Geometry check sheet. Reference: the model listing, model coordinates, mm. A direction names the side the tool comes from. Coordinates: 2 decimals unless noted, no trailing zeros. Write each loop counter-clockwise with the first axis right and the second up, starting at its lowest first coordinate (ties: lowest second). Pieces come first, ordered by that corner, then holes. Notation, with made-up numbers: (-35, 54) -> (16, 54) arc R21 ccw to (16, 91) -> close; hole circle Ø7 at (-36.5, 59.5). An arc over 180 degrees is marked (long way). Answer in a Markdown table with one row per item. Add a question column.
1. Set-up check for faces 4 (the cylindrical face through (-4.769, 7.888, -21.477)), 5 (the cylindrical face through (35.405, 47.707, -13.399)), 6 (the cylindrical face through (35.85, 45.21, -15.5)), 7 (the flat face through (38, 53, 14)): record each of +Z, -Z, +X, -X, +Y, -Y from which the full face is reachable in a straight line by a thin tool's end or side.
2. Cross-section at D-D on y = 68. Record the cut outline in (x, z), and give its area (3 significant figures).
3. Scan lines: L1, parallel to Y at x = 36, z = 31; L2, parallel to Z at x = 0, y = 18; L3, parallel to Y at x = -19, z = -1. Record each from-to range of solid material in increasing order. Write a range as from..to.
4. Mould release check, pull along X, two halves, no side actions. Record for faces 1 (the conical face through (-26.848, 33.914, 1.182)), 2 (the flat face through (39, 53, 17)), 3 (the flat face through (36.6, 46.6, 0.2)): pulls with the +X half, pulls with the -X half, needs draft (parallel to the pull), parting line crosses it, or undercut.
5. Cross-section at A-A on x = 0. Give the number of separate pieces and of enclosed holes in the cut face, and give its area (3 significant figures).
6. Depth check by flat-ended pin: P1, Ø6, axis at x = 34.5, y = 52, coming from the -Z side; P2, Ø5.5, axis at x = 36.5, y = 51, coming from the -Z side; P3, Ø1.5, axis at y = 59, z = -27, coming from the +X side; P4, Ø5, axis at x = -14, z = 0, coming from the -Y side. Enter the tip coordinate at first touch or a pass-through.
```python
from build123d import *

# Parameters (mm, degrees)
F2_R     = 6
F3_DEPTH = 72.001
F2_R_2   = 3
F4_DEPTH = 72.001
F7_DEPTH = 12.5
F8_DEPTH = 8


with BuildPart() as f1:
    # F0 (on Top) → F1 (revolve)
    with BuildSketch(Plane.XY):
        with BuildLine():
            ThreePointArc((26, 0), (33.069705, 39.16163), (53.386308, 73.37931))
            ThreePointArc((53.386308, 73.37931), (54.003261, 77.66091), (50.364391, 80))
            Line((50.364391, 80), (48, 80))
            Line((48, 80), (48, 88))
            Line((48, 88), (40, 88))
            Line((40, 88), (40, 66))
            Line((40, 66), (22, 22))
            Line((22, 22), (0, 22))
            Line((0, 22), (0, 16))
            Line((0, 16), (22, 16))
            Line((22, 16), (22, 0))
            Line((22, 0), (26, 0))
        make_face()
    revolve(axis=Axis((0, 5.929412, 0), (0, -1, 0)))

    # F2 (on face) → F3 (cut, through all)
    with BuildSketch(Plane.XZ.offset(-16)):
        Circle(F2_R)
    extrude(amount=-F3_DEPTH, mode=Mode.SUBTRACT)

    # F2 (on face) → F4 (cut, through all)
    with BuildSketch(Plane.XZ.offset(-16)):
        with Locations((-14, 0)):
            Circle(F2_R_2)
        with Locations((0, 14)):
            Circle(F2_R_2)
        with Locations((14, 0)):
            Circle(F2_R_2)
        with Locations((0, -14)):
            Circle(F2_R_2)
    extrude(amount=-F4_DEPTH, mode=Mode.SUBTRACT)

    # F6 (on face) → F7 (cut, symmetric)
    with BuildSketch(Plane(origin=(11.136283, -4.555752, 0), x_dir=(0.378633, 0.925547, 0), z_dir=(0.925547, -0.378633, 0))):
        with BuildLine():
            ThreePointArc((69.990086, 12), (69.4043, 13.414214), (67.990086, 14))
            Line((67.990086, 14), (58.990086, 14))
            ThreePointArc((58.990086, 14), (57.575873, 13.414214), (56.990086, 12))
            Line((56.990086, 12), (56.990086, -12))
            ThreePointArc((56.990086, -12), (57.575873, -13.414214), (58.990086, -14))
            Line((58.990086, -14), (67.990086, -14))
            ThreePointArc((67.990086, -14), (69.4043, -13.414214), (69.990086, -12))
            Line((69.990086, -12), (69.990086, 12))
        make_face()
    extrude(amount=F7_DEPTH, both=True, mode=Mode.SUBTRACT)

    # F6 (on face) → F8 (join)
    with BuildSketch(Plane(origin=(11.136283, -4.555752, 0), x_dir=(0.378633, 0.925547, 0), z_dir=(0.925547, -0.378633, 0))):
        with BuildLine():
            ThreePointArc((72.990086, 12), (71.52562, 15.535534), (67.990086, 17))
            Line((67.990086, 17), (58.990086, 17))
            ThreePointArc((58.990086, 17), (55.454552, 15.535534), (53.990086, 12))
            Line((53.990086, 12), (53.990086, -12))
            ThreePointArc((53.990086, -12), (55.454552, -15.535534), (58.990086, -17))
            Line((58.990086, -17), (67.990086, -17))
            ThreePointArc((67.990086, -17), (71.52562, -15.535534), (72.990086, -12))
            Line((72.990086, -12), (72.990086, 12))
        make_face()
        with BuildLine():
            Line((58.990086, 14), (67.990086, 14))
            ThreePointArc((67.990086, 14), (69.4043, 13.414214), (69.990086, 12))
            Line((69.990086, 12), (69.990086, -12))
            ThreePointArc((69.990086, -12), (69.4043, -13.414214), (67.990086, -14))
            Line((67.990086, -14), (58.990086, -14))
            ThreePointArc((58.990086, -14), (57.575873, -13.414214), (56.990086, -12))
            Line((56.990086, -12), (56.990086, 12))
            ThreePointArc((56.990086, 12), (57.575873, 13.414214), (58.990086, 14))
        make_face(mode=Mode.SUBTRACT)
    extrude(amount=F8_DEPTH)


solid = f1.part
```
Results found:
| question | item | result |
|---|---|---|
| 1 | face 4 | -Y |
| 1 | face 5 | +X |
| 1 | face 6 | -Z, -Y |
| 1 | face 7 | none |
| 2 | outline | circle Ø98.01 at (0, 0); hole circle Ø80 at (0, 0) |
| 2 | area | 2,520 mm^2 |
| 3 | L1 | y = 65.99..88 |
| 3 | L2 | z = -27.46..-17, -11..-6, 6..11, 17..27.46 |
| 3 | L3 | y = 16..22 |
| 4 | face 1 | undercut |
| 4 | face 2 | needs draft |
| 4 | face 3 | pulls with the +X half |
| 5 | separate pieces | 4 |
| 5 | enclosed holes | 0 |
| 5 | area | 1,230 mm^2 |
| 6 | P1 | stops at z = -23.48 |
| 6 | P2 | stops at z = -18.9 |
| 6 | P3 | stops at x = 34.05 |
| 6 | P4 | passes through |
